```python
from build123d import *

# Parameters (mm, degrees)
SKETCH1_W                = 35
SKETCH1_H                = 26
SKETCH1_R                = 0.925
BOSS_EXTRUDE1_DEPTH      = 3
SKETCH2_R                = 1.389029916
CUT_EXTRUDE4_DEPTH       = 1.5
SKETCH3_W                = 41
SKETCH3_H                = 32
SKETCH3_W_2              = 35
SKETCH3_H_2              = 26
BOSS_EXTRUDE2_DEPTH      = 25
BOSS_EXTRUDE2_DEPTH_BACK = 3
SKETCH4_W                = 18
SKETCH4_H                = 5.71
CUT_EXTRUDE5_DEPTH       = 25
SKETCH5_W                = 9
SKETCH5_H                = 5.71
CUT_EXTRUDE6_DEPTH       = 25
SKETCH6_W                = 3
SKETCH6_H                = 3
CUT_EXTRUDE7_DEPTH       = 25
SKETCH8_W                = 7
SKETCH8_H                = 8
CUT_EXTRUDE8_DEPTH       = 25
SKETCH9_W                = 8
SKETCH9_H                = 3
BOSS_EXTRUDE3_DEPTH      = 5
SKETCH10_W               = 8
SKETCH10_H               = 3
BOSS_EXTRUDE4_DEPTH      = 5
SKETCH11_R               = 0.925
CUT_EXTRUDE9_DEPTH       = 5
SKETCH12_R               = 1.75
CUT_EXTRUDE10_DEPTH      = 1.5
SKETCH13_W               = 8
SKETCH13_H               = 3
BOSS_EXTRUDE5_DEPTH      = 5
SKETCH14_W               = 8
SKETCH14_H               = 3
BOSS_EXTRUDE6_DEPTH      = 5
SKETCH15_R               = 0.925
CUT_EXTRUDE11_DEPTH      = 5
SKETCH17_R               = 1.75
CUT_EXTRUDE13_DEPTH      = 1.5


with BuildPart() as part:
    # Sketch1 → Boss-Extrude1 (new body)
    with BuildSketch(Plane(origin=(0, 0, 0), x_dir=(1, 0, 0), z_dir=(0, 1, 0))):
        with Locations((9.357103431, 0.985655738)):
            Rectangle(SKETCH1_W, SKETCH1_H)
        with Locations((0.557103431, -10.236344262)):
            Circle(SKETCH1_R, mode=Mode.SUBTRACT)
        with Locations((15.924103431, -10.236344262)):
            Circle(SKETCH1_R, mode=Mode.SUBTRACT)
        with Locations((15.924103431, 11.607655738)):
            Circle(SKETCH1_R, mode=Mode.SUBTRACT)
    extrude(amount=BOSS_EXTRUDE1_DEPTH)

    # Sketch2 → Cut-Extrude4 (cut)
    with BuildSketch(Plane.XZ):
        with Locations((0.557103431, 10.236344262)):
            Circle(SKETCH2_R)
        with Locations((15.924103431, 10.236344262)):
            Circle(SKETCH2_R)
        with Locations((15.924103431, -11.607655738)):
            Circle(SKETCH2_R)
    extrude(amount=-CUT_EXTRUDE4_DEPTH, mode=Mode.SUBTRACT)

    # Sketch3 → Boss-Extrude2 (add, two sides)
    with BuildSketch(Plane(origin=(0, 3, 0), x_dir=(1, 0, 0), z_dir=(0, 1, 0))) as boss_extrude2_sk:
        with Locations((9.357103431, 0.985655738)):
            Rectangle(SKETCH3_W, SKETCH3_H)
        with Locations((9.357103431, 0.985655738)):
            Rectangle(SKETCH3_W_2, SKETCH3_H_2, mode=Mode.SUBTRACT)
    extrude(amount=BOSS_EXTRUDE2_DEPTH)
    extrude(boss_extrude2_sk.sketch, amount=-BOSS_EXTRUDE2_DEPTH_BACK)

    # Sketch4 → Cut-Extrude5 (cut)
    with BuildSketch(Plane(origin=(-8.142896569, 0, 0), x_dir=(0, 0, -1), z_dir=(1, 0, 0))):
        with Locations((4.985655738, 25.145)):
            Rectangle(SKETCH4_W, SKETCH4_H)
    extrude(amount=-CUT_EXTRUDE5_DEPTH, mode=Mode.SUBTRACT)

    # Sketch5 → Cut-Extrude6 (cut)
    with BuildSketch(Plane.ZY.offset(-26.857103431)):
        with Locations((-4.985655738, 25.145)):
            Rectangle(SKETCH5_W, SKETCH5_H)
    extrude(amount=-CUT_EXTRUDE6_DEPTH, mode=Mode.SUBTRACT)

    # Sketch6 → Cut-Extrude7 (cut)
    with BuildSketch(Plane(origin=(0, 3, 0), x_dir=(1, 0, 0), z_dir=(0, 1, 0))):
        with Locations((0.68611622, -7.236344262)):
            Rectangle(SKETCH6_W, SKETCH6_H)
    extrude(amount=-CUT_EXTRUDE7_DEPTH, mode=Mode.SUBTRACT)

    # Sketch8 → Cut-Extrude8 (cut)
    with BuildSketch(Plane.XY.offset(15.014344262)):
        with Locations((20.765233628, 9.653180084)):
            Rectangle(SKETCH8_W, SKETCH8_H)
    extrude(amount=-CUT_EXTRUDE8_DEPTH, mode=Mode.SUBTRACT)

    # Sketch9 → Boss-Extrude3 (add)
    with BuildSketch(Plane(origin=(0, 0, -16.985655738), x_dir=(-1, 0, 0), z_dir=(0, 0, -1))):
        with Locations((7.142896569, 1.5)):
            Rectangle(SKETCH9_W, SKETCH9_H)
        with Locations((-25.857103431, 1.5)):
            Rectangle(SKETCH9_W, SKETCH9_H)
    extrude(amount=BOSS_EXTRUDE3_DEPTH)

    # Sketch10 → Boss-Extrude4 (add)
    with BuildSketch(Plane.XY.offset(15.014344262)):
        with Locations((-7.142896569, 1.5)):
            Rectangle(SKETCH10_W, SKETCH10_H)
        with Locations((25.857103431, 1.5)):
            Rectangle(SKETCH10_W, SKETCH10_H)
    extrude(amount=BOSS_EXTRUDE4_DEPTH)

    # Sketch11 → Cut-Extrude9 (cut)
    with BuildSketch(Plane(origin=(0, 3, 0), x_dir=(1, 0, 0), z_dir=(0, 1, 0))):
        with Locations((-7.142896569, -17.514344262)):
            Circle(SKETCH11_R)
        with Locations((25.857103431, -17.514344262)):
            Circle(SKETCH11_R)
        with Locations((25.857103431, 19.485655738)):
            Circle(SKETCH11_R)
        with Locations((-7.142896569, 19.485655738)):
            Circle(SKETCH11_R)
    extrude(amount=-CUT_EXTRUDE9_DEPTH, mode=Mode.SUBTRACT)

    # Sketch12 → Cut-Extrude10 (cut)
    with BuildSketch(Plane(origin=(0, 3, 0), x_dir=(1, 0, 0), z_dir=(0, 1, 0))):
        with Locations((-7.142896569, -17.514344262)):
            Circle(SKETCH12_R)
        with Locations((-7.142896569, 19.485655738)):
            Circle(SKETCH12_R)
        with Locations((25.857103431, 19.485655738)):
            Circle(SKETCH12_R)
        with Locations((25.857103431, -17.514344262)):
            Circle(SKETCH12_R)
    extrude(amount=-CUT_EXTRUDE10_DEPTH, mode=Mode.SUBTRACT)

    # Sketch13 → Boss-Extrude5 (add)
    with BuildSketch(Plane.XY.offset(15.014344262)):
        with Locations((25.857103431, 26.5)):
            Rectangle(SKETCH13_W, SKETCH13_H)
        with Locations((-7.142896569, 26.5)):
            Rectangle(SKETCH13_W, SKETCH13_H)
    extrude(amount=BOSS_EXTRUDE5_DEPTH)

    # Sketch14 → Boss-Extrude6 (add)
    with BuildSketch(Plane(origin=(0, 0, -16.985655738), x_dir=(-1, 0, 0), z_dir=(0, 0, -1))):
        with Locations((-25.857103431, 26.5)):
            Rectangle(SKETCH14_W, SKETCH14_H)
        with Locations((7.142896569, 26.5)):
            Rectangle(SKETCH14_W, SKETCH14_H)
    extrude(amount=BOSS_EXTRUDE6_DEPTH)

    # Sketch15 → Cut-Extrude11 (cut)
    with BuildSketch(Plane.XZ.offset(-25)):
        with Locations((25.857103431, 17.514344262)):
            Circle(SKETCH15_R)
        with Locations((-7.142896569, 17.514344262)):
            Circle(SKETCH15_R)
        with Locations((25.857103431, -19.485655738)):
            Circle(SKETCH15_R)
        with Locations((-7.142896569, -19.485655738)):
            Circle(SKETCH15_R)
    extrude(amount=-CUT_EXTRUDE11_DEPTH, mode=Mode.SUBTRACT)

    # Sketch17 → Cut-Extrude13 (cut)
    with BuildSketch(Plane.XZ.offset(-25)):
        with Locations((25.857103431, -19.485655738)):
            Circle(SKETCH17_R)
        with Locations((25.857103431, 17.514344262)):
            Circle(SKETCH17_R)
        with Locations((-7.142896569, 17.514344262)):
            Circle(SKETCH17_R)
        with Locations((-7.142896569, -19.485655738)):
            Circle(SKETCH17_R)
    extrude(amount=-CUT_EXTRUDE13_DEPTH, mode=Mode.SUBTRACT)


solid = part.part
```
The listing builds one solid part. Answer for the finished solid, in the listing's coordinates (mm). A direction names the side the tool comes from. Give positions to 0.01 mm unless a question says otherwise; leave off trailing zeros. Loops run counter-clockwise (first coordinate to the right, second up) from the corner with the lowest first, then second, coordinate; pieces in that order, holes last. Notation, with made-up numbers: (36.5, 0.5) - (81.5, 0.5) arc R29 ccw to (81.5, 33.5) - close; hole circle Ø10 at (25, 15.25). An arc over 180 degrees is marked (long way). Answer as CSV lines item,"result". Start each with the question number.
Item 1: Each of these flat-tipped pins is pushed along its axis until it touches: pin 1 (3 mm diameter, centred on x = 2, y = 6, fed in from +Z); pin 2 (5 mm diameter, centred on x = -5, y = 9.5, fed in from -Z); pin 3 (0.9 mm diameter, centred on x = -10, z = -2, fed in from +Y); pin 4 (1.5 mm diameter, centred on x = -7.14, z = -19.49, fed in from +Y). Where does it stop, or does it pass through?
Item 2: The mould has two halves that part along Z. Classify faces 1 (the face through (-6, 26.5, 17)), 2 (the face through (29.857, 14, -1)), 3 (the face through (9, 14, -16.986)), 4 (the face through (9, 14, 15.014)): +Z half, -Z half, draft (parallel to the pull), parting line (faces both ways), or undercut.
Item 3: Find the intervals of material crossed by line 1 (Z direction, x = 23.5, y = 23.5); line 2 (X direction, y = 23, z = 7); line 3 (Y direction, x = 25.5, z = 2.5), in increasing order. Write a range as from..to.
Item 4: A cutting plane is placed at D-D on z = 2. Determine the outline of the cut face in (x, y), then the cut area to 3 significant figures.
Item 5: A cutting plane is placed at C-C on x = 21. Determine the outline of the cut face in (y, z).
Item 6: A cutting plane is placed at A-A on y = 21.75. Determine the outline of the cut face in (x, z).
Item 7: A cutting plane is placed at B-B on z = 13.5. Determine the outline of the cut face in (x, y).
Item 8: For faces 5 (the face through (28, 25, -0.486)), 6 (the face through (24, 25, 17)), 7 (the face through (-0.814, 2, 7)), 8 (the face through (27, 26.5, -20)), determine the directions among +Z, -Z, +X, -X, +Y, -Y from which every point of the face is accessible in a straight line to the end or side of a thin tool.
Found:
1,pin 1,"stops at z = 15.01"
1,pin 2,"stops at z = -16.99"
1,pin 3,"stops at y = 22.29"
1,pin 4,"passes through"
2,face 1,"undercut"
2,face 2,"draft"
2,face 3,"-Z half"
2,face 4,"+Z half"
3,line 1,"z = -16.99..-13.99, 12.01..15.01"
3,line 2,"x = -11.14..-8.14, 26.86..29.86"
3,line 3,"y = 0..3"
4,outline,"(-11.14, 0) - (29.86, 0) - (29.86, 28) - (26.86, 28) - (26.86, 3) - (-8.14, 3) - (-8.14, 22.29) - (-11.14, 22.29) - close"
4,area,"256 mm^2"
5,outline,"(0, -16.99) - (28, -16.99) - (28, -13.99) - (3, -13.99) - (3, 12.01) - (5.65, 12.01) - (5.65, 15.01) - (0, 15.01) - close; (13.65, 12.01) - (28, 12.01) - (28, 15.01) - (13.65, 15.01) - close"
6,outline,"(-11.14, -16.99) - (29.86, -16.99) - (29.86, 15.01) - (-11.14, 15.01) - close; hole (-8.14, -13.99) - (26.86, -13.99) - (26.86, 12.01) - (-8.14, 12.01) - close"
7,outline,"(-11.14, 0) - (29.86, 0) - (29.86, 28) - (-11.14, 28) - close; hole (17.27, 5.65) - (24.27, 5.65) - (24.27, 13.65) - (17.27, 13.65) - close"
8,face 5,"+X, -X, +Y"
8,face 6,"+Z, +X, -X"
8,face 7,"+Y, -Y"
8,face 8,"none"
